from build123d import *

# Parameters (mm, degrees)
SKETCH_1_R                       = 1.5
SKETCH_1_R_2                     = 12
SM_BASE_FLANGE_1_DEPTH           = 1.5
SM_EDGE_FLANGE_1_STRIP_W         = 8
SM_EDGE_FLANGE_1_STRIP_H         = 1.5
SM_EDGE_FLANGE_1_STRIP_CUT_DEPTH = 40
SM_EDGE_FLANGE_1_DEPTH           = 40
SM_EDGE_FLANGE_1_PROFILE_R       = 2
SM_EDGE_FLANGE_1_FLAT_DEPTH      = 1.5


# Sheet-metal steps are written as plain solids
with BuildPart() as part:
    # Sketch 1 → 基体-法兰1 (new body)
    with BuildSketch(Plane.XY):
        with BuildLine():
            Line((-20, 21.5), (20, 21.5))
            Line((20, 21.5), (20, -18))
            ThreePointArc((20, -18), (19.121320344, -20.121320344), (17, -21))
            Line((17, -21), (-17, -21))
            ThreePointArc((-17, -21), (-19.121320344, -20.121320344), (-20, -18))
            Line((-20, -18), (-20, 21.5))
        make_face()
        with Locations((-15.5, 15.5)):
            Circle(SKETCH_1_R, mode=Mode.SUBTRACT)
        with Locations(Location((15.5, 15.5, 0), (0, 0, 180))):
            Circle(SKETCH_1_R, mode=Mode.SUBTRACT)
        with Locations((15.5, -15.5)):
            Circle(SKETCH_1_R, mode=Mode.SUBTRACT)
        with Locations(Location((-15.5, -15.5, 0), (0, 0, 180))):
            Circle(SKETCH_1_R, mode=Mode.SUBTRACT)
        Circle(SKETCH_1_R_2, mode=Mode.SUBTRACT)
    extrude(amount=-SM_BASE_FLANGE_1_DEPTH)

    # 边线-法兰1 strip (across the edge) → 边线-法兰1 strip cut (cut)
    with BuildSketch(Plane(origin=(20, 21.5, 0), x_dir=(0, -1, 0), z_dir=(-1, 0, 0))):
        with Locations((-1.5, -0.75)):
            Rectangle(SM_EDGE_FLANGE_1_STRIP_W, SM_EDGE_FLANGE_1_STRIP_H)
    extrude(amount=SM_EDGE_FLANGE_1_STRIP_CUT_DEPTH, mode=Mode.SUBTRACT)

    # 边线-法兰1 bend section (across the edge) → 边线-法兰1 (add)
    with BuildSketch(Plane(origin=(20, 21.5, 0), x_dir=(0, -1, 0), z_dir=(-1, 0, 0))):
        with BuildLine():
            Line((0, 1), (1.5, 1))
            ThreePointArc((1.5, 1), (1.792893219, 0.292893219), (2.5, 0))
            Line((2.5, 0), (2.5, -1.5))
            ThreePointArc((2.5, -1.5), (0.732233047, -0.767766953), (0, 1))
        make_face()
    extrude(amount=SM_EDGE_FLANGE_1_DEPTH)

    # 边线-法兰1 profile (on flange) → 边线-法兰1 flat (add)
    with BuildSketch(Plane(origin=(0, 21.5, 0), x_dir=(-1, 0, 0), z_dir=(0, 1, 0))):
        with BuildLine():
            Line((15, 14.5), (-15, 14.5))
            ThreePointArc((-15, 14.5), (-18.535533906, 13.035533906), (-20, 9.5))
            Line((-20, 9.5), (-20, 1))
            Line((-20, 1), (20, 1))
            Line((20, 1), (20, 9.5))
            ThreePointArc((20, 9.5), (18.535533906, 13.035533906), (15, 14.5))
        make_face()
        with Locations((-10, 7)):
            Circle(SM_EDGE_FLANGE_1_PROFILE_R, mode=Mode.SUBTRACT)
        with Locations((10, 7)):
            Circle(SM_EDGE_FLANGE_1_PROFILE_R, mode=Mode.SUBTRACT)
    extrude(amount=-SM_EDGE_FLANGE_1_FLAT_DEPTH)


solid = part.part
Build history of the part. All positions in model axes, mm. A direction names the side the tool comes from. Give positions to 0.01 mm unless a question says otherwise; leave off trailing zeros. Order: outer loops, then holes, each group sorted by start corner. A loop starts at its lowest first (then second) coordinate and runs counter-clockwise, first axis right, second up. Notation, with made-up numbers: M 65,67 L 88,67 A14 ccw 88,83 Z; hole C -24,37 d10. An arc over 180 degrees is marked long. Use one line per item in the form item = value.
Q1. Slice it at A-A, the plane x = 0. Write the cut outline in (y, z), and give its area (3 significant figures).
Conclusion:
outline = M -21,-1.5 L -12,-1.5 L -12,0 L -21,0 Z; M 12,-1.5 L 19,-1.5 A2.5 ccw 21.5,1 L 21.5,14.5 L 20,14.5 L 20,1 A1 cw 19,0 L 12,0 Z
area = 48.4 mm2
Q2. Slice it at B-B, the plane y = 15.5. Write the cut outline in (x, z).
Conclusion:
outline = M -20,-1.5 L -17,-1.5 L -17,0 L -20,0 Z; M -14,-1.5 L 14,-1.5 L 14,0 L -14,0 Z; M 17,-1.5 L 20,-1.5 L 20,0 L 17,0 Z
Q3. Which spindle directions (+Z, -Z, +X, -X, +Y, -Y) get a long thin tool onto all of the face, cutting with end or side? Do faces 5 (the flat face through (0, 20, 8)), 6 (the cylindrical face through (0.28, 20.748, -0.787)). Say none if no direction does.
Conclusion:
face_5 = +Z, +X, -X, -Y
face_6 = -Z, +X, -X, +Y
Q4. Pull direction X, two halves, no side cores. Call faces 1 (the cylindrical face through (-11.99, 0.53, -0.74)), 2 (the flat face through (20, 5, -1)), 3 (the cylindrical face through (0.28, 19.715, 0.301)), 4 (the cylindrical face through (-17, 15.57, -0.74)): released by +X, released by -X, zero draft, split by the parting line, or undercut.
Conclusion:
face_1 = undercut
face_2 = released by +X
face_3 = zero draft
face_4 = undercut
Q5. Slice it at C-C, the plane z = 7. Write the cut outline in (x, y).
Conclusion:
outline = M -20,20 L -12,20 L -12,21.5 L -20,21.5 Z; M -8,20 L 8,20 L 8,21.5 L -8,21.5 Z; M 12,20 L 20,20 L 20,21.5 L 12,21.5 Z
Q6. Pin check, flat tips, straight feed: P1, Ø4, axis at x = -1, z = 9, coming from the -Y side; P2, Ø12, axis at x = 0, y = 9, coming from the -Z side; P3, Ø20, axis at x = 7, y = 3, coming from the +Z side; P4, Ø2.5, axis at x = -15.5, y = -15.5, coming from the -Z side. Stop position of each tip, or through.
Conclusion:
P1 = 20
P2 = -1.5
P3 = 0
P4 = through
Q7. Slice it at D-D, the plane x = -15.5. Write the cut outline in (y, z), and give its area (3 significant figures).
Conclusion:
outline = M -21,-1.5 L -17,-1.5 L -17,0 L -21,0 Z; M -14,-1.5 L 14,-1.5 L 14,0 L -14,0 Z; M 17,-1.5 L 19,-1.5 A2.5 ccw 21.5,1 L 21.5,14.47 L 20,14.47 L 20,1 A1 cw 19,0 L 17,0 Z
area = 75.3 mm2
Q8. Wall check: probe 1 along Y at (x, z) = (15.5, -0.85); probe 2 along Y at (x, z) = (-15.5, -0.3); probe 3 along Z at (x, y) = (13.5, 16). Give the ranges that are in metal, low to high.
Conclusion:
probe_1 = -21 to -17, -14 to 14, 17 to 20.68
probe_2 = -21 to -17, -14 to 14, 17 to 21.14
probe_3 = -1.5 to 0
